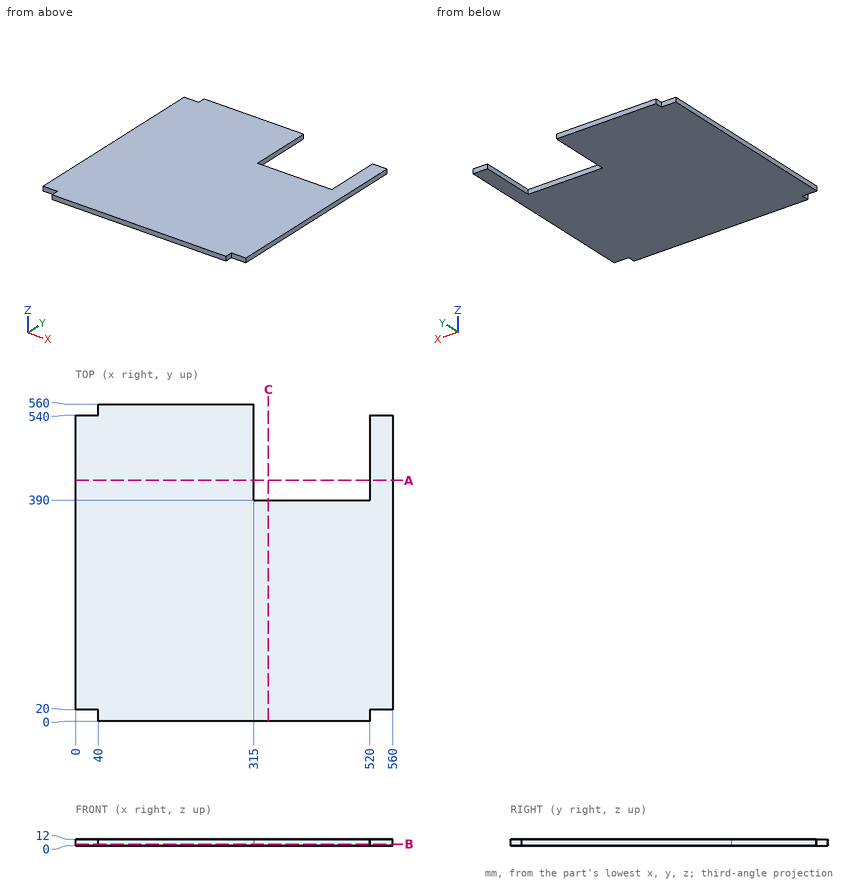
The drawing under review shows one solid part. Ordinate dimensions are in mm from its lowest x, y, z. Coordinates: 2 decimals unless noted, no trailing zeros. Write each loop counter-clockwise with the first axis right and the second up, starting at its lowest first coordinate (ties: lowest second). Pieces come first, ordered by that corner, then holes. Notation, with made-up numbers: M -3.5,76 L 15.5,76 A27 cw 15.5,104 Z; hole C 63.5,31 d10. An arc over 180 degrees is marked long. Put each result on its own line as item: value.
1) Add section A-A on y = 425. Give the boundary of the cut face in (x, z).
Computed:
outline: M 0,0 L 315,0 L 315,12 L 0,12 Z; M 520,0 L 560,0 L 560,12 L 520,12 Z
2) Clearance check with flat-ended pins moving along their axes: pin 1 Ø6 at (x, z) = (24.5, 6) entering from -Y; pin 2 Ø6 at (x, z) = (27, 3.5) entering from +Y; pin 3 Ø6 at (x, z) = (377.5, 8) entering from +Y. State where each tip first meets the part, or that it passes through.
Computed:
pin 1: stops at y = 20
pin 2: stops at y = 540
pin 3: stops at y = 390
3) Add section C-C on x = 340.5. Give the boundary of the cut face in (y, z).
Computed:
outline: M 0,0 L 390,0 L 390,12 L 0,12 Z
4) Wall thickness on probe 1 along X at (y, z) = (458, 6.5); probe 2 along Y at (x, z) = (536, 6.75); probe 3 along Y at (x, z) = (424, 3.25): over which ranges is each line inside the solid? List them lowest first. Write a range as [from, to].
Computed:
probe 1: x = [0, 315], [520, 560]
probe 2: y = [20, 540]
probe 3: y = [0, 390]
5) Add section B-B on z = 2.75. Give the boundary of the cut face in (x, y).
Computed:
outline: M 0,20 L 40,20 L 40,0 L 520,0 L 520,20 L 560,20 L 560,540 L 520,540 L 520,390 L 315,390 L 315,560 L 40,560 L 40,540 L 0,540 Z
